Design review of the part shown in the three views and the two pictorial views. Dimensions are in mm from the part's minimum x, y and z. A direction names the side the tool comes from. Give positions to 0.01 mm unless a question says otherwise; leave off trailing zeros. Loops run counter-clockwise (first coordinate to the right, second up) from the corner with the lowest first, then second, coordinate; pieces in that order, holes last. Notation, with made-up numbers: (57, 22.25) - (93, 22.25) arc R21 cw to (93, 41.25) - close; hole circle Ø8 at (49.5, 65). An arc over 180 degrees is marked (long way). Answer as a JSON object with one key per item and string values.
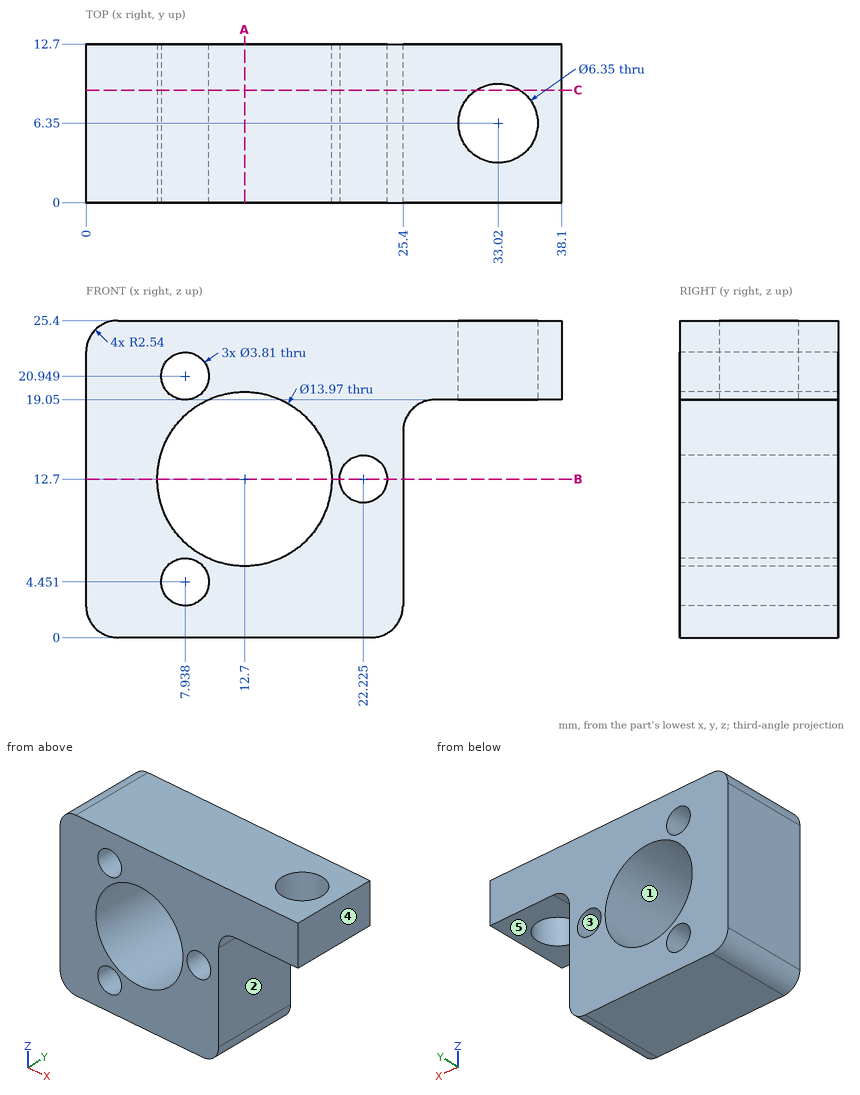
Q1. Consider section B-B, the plane z = 12.7. State the section outline as (x, y) points (1 decimal).
Results:
{"outline": "(0, 0) - (5.7, 0) - (5.7, 12.7) - (0, 12.7) - close; (19.7, 0) - (20.3, 0) - (20.3, 12.7) - (19.7, 12.7) - close; (24.1, 0) - (25.4, 0) - (25.4, 12.7) - (24.1, 12.7) - close"}
Q2. Consider section A-A, the plane x = 12.7. State the section outline as (y, z) points (1 decimal).
Results:
{"outline": "(0, 0) - (12.7, 0) - (12.7, 5.7) - (0, 5.7) - close; (0, 19.7) - (12.7, 19.7) - (12.7, 25.4) - (0, 25.4) - close"}
Q3. Clearance check with a flat-ended pin moving along its axis: pin 1 Ø1.5 at (y, z) = (8.5, 7.5) entering from +X. State where the tip first meets the part, or that it passes through.
Results:
{"pin 1": "stops at x = 25.4"}
Q4. For the marked faces 1 and 2, list the 3-axis set-ups (+Z, -Z, +X, -X, +Y, -Y) from which the entire face can be reached by the end or side of a thin tool; tool diameter is ignored.
Results:
{"face 1": "+Y, -Y", "face 2": "-Z, +X, +Y, -Y"}
Q5. Consider section C-C, the plane y = 9. State how many separate pieces and enclosed holes the cut face has.
Results:
{"separate pieces": "2", "enclosed holes": "4"}
Q6. To check wall thickness, follow probe 1 along X at (y, z) = (5.25, 12.7) (1 decimal); probe 2 along Y at (x, z) = (33.02, 23) (1 decimal); probe 3 along Z at (x, y) = (9.5, 7.25) (1 decimal). State the ranges of each line that lie inside material, in increasing order. Write a range as [from, to].
Results:
{"probe 1": "x = [0, 5.7], [19.7, 20.3], [24.1, 25.4]", "probe 2": "y = [0, 3.2], [9.5, 12.7]", "probe 3": "z = [0, 3.4], [5.5, 6.5], [18.9, 19.9], [22, 25.4]"}
Q7. The part is to be moulded in two halves that separate along Z. For the marked faces 3, 4 and 5, say which applies: +Z half, -Z half, draft (parallel to the pull), parting line (faces both ways), or undercut.
Results:
{"face 3": "undercut", "face 4": "draft", "face 5": "-Z half"}
